from build123d import *

# Parameters (mm, degrees)
SKETCH1_R               = 30
BOSS_EXTRUDE1_DEPTH     = 20
SKETCH2_R               = 6
BOSS_EXTRUDE2_DEPTH     = 5
BOSS_EXTRUDE3_DEPTH     = 2.5
SKETCH8_R               = 3
BOSS_EXTRUDE4_DEPTH     = 3
MIRROR2_COPY_1_DEPTH    = 2.5
SKETCH3_R               = 25
CUT_EXTRUDE1_DEPTH      = 55.706602517
CUT_EXTRUDE1_DEPTH_BACK = 41.0000001
FILLET1_R               = 5


with BuildPart() as part:
    # Sketch1 → Boss-Extrude1 (new body, symmetric)
    with BuildSketch(Plane.XY):
        Circle(SKETCH1_R)
    extrude(amount=BOSS_EXTRUDE1_DEPTH, both=True)

    # Sketch2 → Boss-Extrude2 (add, symmetric)
    with BuildSketch(Plane(origin=(0, 0, 0), x_dir=(0, 0, -1), z_dir=(1, 0, 0))):
        with BuildLine():
            Line((-15, 0), (5, 0))
            Line((5, 0), (5, -89.20774256))
            ThreePointArc((5, -89.20774256), (4.06307787, -93.433925178), (1.427876097, -96.868186992))
            Line((1.427876097, -96.868186992), (-41.654587977, -133.018666706))
            ThreePointArc((-41.654587977, -133.018666706), (-43.886965918, -135.679111138), (-45.07478941, -138.942629361))
            Line((-45.07478941, -138.942629361), (-50.15192247, -167.736481777))
            ThreePointArc((-50.15192247, -167.736481777), (-60, -176), (-69.84807753, -167.736481777))
            Line((-69.84807753, -167.736481777), (-74.554680047, -141.044012488))
            ThreePointArc((-74.554680047, -141.044012488), (-74.103528725, -135.887329278), (-71.134478614, -131.64708628))
            Line((-71.134478614, -131.64708628), (-18.572123903, -87.542033829))
            ThreePointArc((-18.572123903, -87.542033829), (-15.93692213, -84.107772015), (-15, -79.881589397))
            Line((-15, -79.881589397), (-15, 0))
        make_face()
        with Locations((-60, -166)):
            Circle(SKETCH2_R, mode=Mode.SUBTRACT)
    extrude(amount=BOSS_EXTRUDE2_DEPTH, both=True)

    # Sketch5 → Boss-Extrude3 (add, symmetric)
    with BuildSketch(Plane(origin=(0, -10, 10), x_dir=(1, 0, 0), z_dir=(0, 1, 0))):
        with BuildLine():
            Line((60.980762114, -15), (70, -15))
            Line((70, -15), (70, -40))
            Line((70, -40), (51, -40))
            ThreePointArc((51, -40), (32.615223689, -32.384776311), (25, -14))
            Line((25, -14), (25, 10))
            ThreePointArc((25, 10), (49.835639165, 7.351904144), (60.980762114, -15))
        make_face()
    boss_extrude3 = extrude(amount=BOSS_EXTRUDE3_DEPTH, both=True)

    # Mirror1: Boss-Extrude3 across plane
    add(boss_extrude3.mirror(Plane.ZX))

    # Sketch7 → Revolve1 (revolve)
    with BuildSketch(Plane.XZ, mode=Mode.PRIVATE) as revolve1_sk:
        with BuildLine():
            Line((70, 17.5), (80, 17.5))
            Line((80, 17.5), (80, 25))
            Line((80, 25), (87, 25))
            Line((87, 25), (87, 32.5))
            Line((87, 32.5), (107, 32.5))
            ThreePointArc((107, 32.5), (117.095800854, 28.88751392), (123.483314774, 37.5))
            Line((123.483314774, 37.5), (70, 37.5))
            Line((70, 37.5), (70, 17.5))
        make_face()
    revolve1 = revolve(revolve1_sk.sketch.rotate(Axis((70, 0, 37.5), (1, 0, 0)), 180), axis=Axis((70, 0, 37.5), (1, 0, 0)))  # turned: the seam where the file's is

    # Sketch8 → Boss-Extrude4 (add, symmetric)
    with BuildSketch(Plane.XY.offset(10)):
        with BuildLine():
            Line((24.859943406, 25.884033957), (21.735901111, 20.677296799))
            ThreePointArc((21.735901111, 20.677296799), (15.434872663, 25.724787771), (8.0160143, 28.909228885))
            Line((8.0160143, 28.909228885), (11.140056594, 34.115966043))
            ThreePointArc((11.140056594, 34.115966043), (22.115966043, 36.859943406), (24.859943406, 25.884033957))
        make_face()
        with Locations((18, 30)):
            Circle(SKETCH8_R, mode=Mode.SUBTRACT)
    boss_extrude4 = extrude(amount=BOSS_EXTRUDE4_DEPTH, both=True)

    # Mirror2: Boss-Extrude4, Revolve1, Boss-Extrude3 across plane
    add(boss_extrude4.mirror(Plane(origin=(0, 0, 0), x_dir=(0, 0, 1), z_dir=(1, 0, 0))))
    add(revolve1.mirror(Plane(origin=(0, 0, 0), x_dir=(0, 0, 1), z_dir=(1, 0, 0))))
    add(boss_extrude3.mirror(Plane(origin=(0, 0, 0), x_dir=(0, 0, 1), z_dir=(1, 0, 0))))

    # Mirror2 copy 1 sketch → Mirror2 copy 1 (add, symmetric)
    with BuildSketch(Plane(origin=(0, 10, 10), x_dir=(-1, 0, 0), z_dir=(0, -1, 0))):
        with BuildLine():
            Line((60.980762114, -15), (70, -15))
            Line((70, -15), (70, -40))
            Line((70, -40), (51, -40))
            ThreePointArc((51, -40), (32.615223689, -32.384776311), (25, -14))
            Line((25, -14), (25, 10))
            ThreePointArc((25, 10), (49.835639165, 7.351904144), (60.980762114, -15))
        make_face()
    extrude(amount=MIRROR2_COPY_1_DEPTH, both=True)

    # Sketch3 → Cut-Extrude1 (cut, two sides)
    with BuildSketch(Plane.XY.offset(20)) as cut_extrude1_sk:
        Circle(SKETCH3_R)
    extrude(amount=CUT_EXTRUDE1_DEPTH, mode=Mode.SUBTRACT)
    extrude(cut_extrude1_sk.sketch, amount=-CUT_EXTRUDE1_DEPTH_BACK, mode=Mode.SUBTRACT)

    # Fillet1
    fillet1_edges = [part.edges().sort_by_distance(p)[0] for p in [
        (-60.980762114, -10, 25),
        (-60.980762114, 10, 25),
        (60.980762114, -10, 25),
        (60.980762114, 10, 25),
    ]]
    fillet(fillet1_edges, radius=FILLET1_R)


solid = part.part
Input: part model. Units: mm. Frame: model coordinates. A direction names the side the tool comes from. Give positions to 0.01 mm unless a question says otherwise; leave off trailing zeros. Loops run counter-clockwise (first coordinate to the right, second up) from the corner with the lowest first, then second, coordinate; pieces in that order, holes last. Notation, with made-up numbers: M 50,84 L 84,84 A11 cw 84,95 Z; hole C 21.5,44 d4. An arc over 180 degrees is marked long. Use one line per item in the form item = value.
1. Section query A-A, the plane y = 0. Count the separate pieces of the cut face and the enclosed holes in it, and give its area (3 significant figures).
Numbers:
separate_pieces = 4
enclosed_holes = 0
area = 2,440 mm²
2. First-contact query: pin 1 (22.5 mm diameter, centred on x = 45, z = 11, fed in from -Y); pin 2 (9.5 mm diameter, centred on x = 18, y = 30, fed in from -Z); pin 3 (1.5 mm diameter, centred on x = -65, y = 9, fed in from +Z). Flat tips, straight axial feed; report the tip coordinate or a pass-through.
Numbers:
pin_1 = -12.5
pin_2 = 7
pin_3 = 50
3. Section query B-B, the plane x = 18. Return the cut outline in (y, z).
Numbers:
outline = M -24,-20 L -17.35,-20 L -17.35,20 L -24,20 Z; M 17.35,-20 L 24,-20 L 24,7 L 27,7 L 27,13 L 24,13 L 24,20 L 17.35,20 Z; M 33,7 L 38,7 L 38,13 L 33,13 Z
4. Reachability of faces 1 (the face through (-75.07, -6.007, 56.576)), 2 (the face through (-32.82, 9.96, 42.59)), 3 (the face through (-97.14, -0.22, 32.505)) from +Z, -Z, +X, -X, +Y, -Y: full face, straight path, thin tool, end or side. Return the list, or none.
Numbers:
face_1 = -X
face_2 = +Z, +Y, -Y
face_3 = none
5. Line query: L1, parallel to Y at x = -49, z = 33.5; L2, parallel to X at y = 11.5, z = 24; L3, parallel to Y at x = -18, z = 8.45. Output: solid intervals per line, ascending.
Numbers:
L1 = -12.5 to -7.5, 7.5 to 12.5
L2 = -80 to -70, -62.74 to -25, 25 to 62.74, 70 to 80
L3 = -24 to -17.35, 17.35 to 27, 33 to 38
6. Pull-direction query (Y, two-part tool) for faces 4 (the face through (32.82, -9.96, 42.59)), 5 (the face through (23.846, 7.509, 0.28)), 6 (the face through (0.07, -154.577, 72.168)), 7 (the face through (-83.549, -0.55, 25.012)); classes: released by +Y, released by -Y, zero draft, split by the parting line, or undercut.
Numbers:
face_4 = zero draft
face_5 = undercut
face_6 = released by -Y
face_7 = split by the parting line
7. Section query D-D, the plane x = -95.5. Return the cut outline in (y, z), and give its area (3 significant figures).
Numbers:
outline = C 0,37.5 d10
area = 78.5 mm²
8. Section query C-C, the plane x = 56.5. Return the cut outline in (y, z), and give its area (3 significant figures).
Numbers:
outline = M -12.5,9.38 L -7.5,9.38 L -7.5,50 L -12.5,50 Z; M 7.5,9.38 L 12.5,9.38 L 12.5,50 L 7.5,50 Z
area = 406 mm²
